Autodesk Inventor part; units mm, degrees
ref_plane "YZ Plane" through (0, 0, 0) normal (1, 0, 0) x (0, 1, 0)
ref_plane "XZ Plane" through (0, 0, 0) normal (0, 1, 0) x (-1, 0, 0)
ref_plane "XY Plane" through (0, 0, 0) normal (0, 0, 1) x (1, 0, 0)
sketch "Sketch1" plane through (0, 0, 0) normal (0, 0, 1) x (1, 0, 0)
  line L0 (-50, 45) -> (50, 45)
  line L1 (50, 45) -> (50, -45)
  line L2 (50, -45) -> (-50, -45)
  line L3 (-50, -45) -> (-50, 45)
  point P0 (0, 0)
  dimension "d0" = 100
  dimension "d1" = 90
  dimension "d2" = 50
  dimension "d3" = 45
extrude "Extrusion1" add sketch "Sketch1" along normal blind 2.6568
fillet "Fillet1" radius 10 4 edges at (50, 45, 1.3284) (-50, 45, 1.3284) (50, -45, 1.3284) (-50, -45, 1.3284)
sketch "Sketch2" plane through (0, 0, 2.6568) normal (0, 0, 1) x (1, 0, 0)
  line L0 (50, 35) -> (50, -35)
  line L1 (-40, 45) -> (40, 45)
  circle A0 centre (40, 32.3) radius 2.75
  circle A1 centre (40, -32.3) radius 3.5685
  point P0 (0, 0)
  dimension "d7" = 5.5
  dimension "d8" = 10
  dimension "d10" = 7.137
  dimension "d12" = 10
  dimension "d52" = 64.6
  dimension "d53" = 12.7
extrude "Extrusion2" cut sketch "Sketch2" against normal through all
pattern_linear "Rectangular Pattern1" count 3 spacing 40 along (-1, 0, 0) of "Extrusion2"
sketch "Sketch3" plane through (0, 0, 2.6568) normal (0, 0, 1) x (1, 0, 0)
  line L0 (40, -45) -> (-40, -45)
  line L1 (-50, -35) -> (-50, 35)
  circle A0 centre (-25, -10) radius 2.6
  point P0 (0, 0)
  dimension "d18" = 5.2
  dimension "d19" = 25
  dimension "d20" = 35
extrude "Extrusion3" cut sketch "Sketch3" against normal through all
pattern_linear "Rectangular Pattern2" count 3 spacing 25 along (1, 0, 0) count 2 spacing 20 along (0, 1, 0) of "Extrusion3"
properties part number "S2SM-01" material "Steel, Mild"
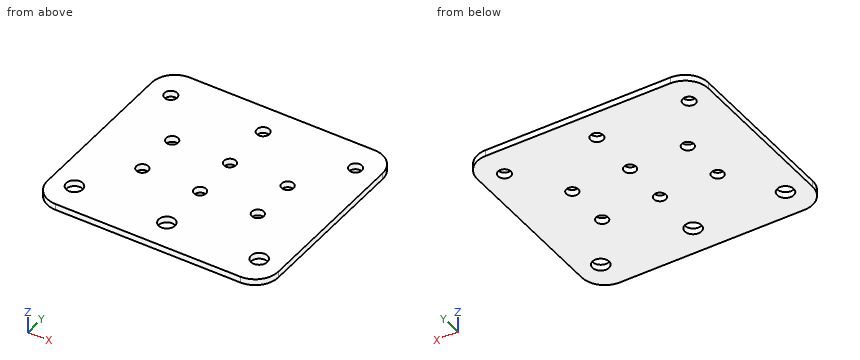
Work out the finished part from the listing and answer in its coordinate system (mm). Give positions to 0.01 mm unless a question says otherwise; leave off trailing zeros. Order: outer loops, then holes, each group sorted by start corner. A loop starts at its lowest first (then second) coordinate and runs counter-clockwise, first axis right, second up.
1. Section C-C, the plane z = 1.1 is taken. Give the number of separate pieces and of enclosed holes in the cut face, and give its area (3 significant figures).
Result sheet:
separate pieces: 1
enclosed holes: 12
area: 8,600 mm2
2. Straight lines are drawn through the part: L1, parallel to Y at x = -40, z = 1; L2, parallel to Y at x = 25, z = 2; L3, parallel to X at y = -35, z = 1.7. For each, find the intervals that lie inside material, in ascending order.
Result sheet:
L1: y = -45 to -35.87, -28.73 to 29.55, 35.05 to 45
L2: y = -45 to -12.6, -7.4 to 7.4, 12.6 to 45
L3: x = -50 to -42.33, -37.67 to -2.33, 2.33 to 37.67, 42.33 to 50
3. This flat-tipped pin is pushed along its axis until it touches: P1, Ø11.5, axis at x = 0, y = -32.3, coming from the -Z side. Where does it stop, or does it pass through?
Result sheet:
P1: stops at z = 0
4. Section D-D, the plane y = 32.3 is taken. Determine the outline of the cut face in (x, z), and give its area (3 significant figures).
Result sheet:
outline: (-50, 0) - (-42.75, 0) - (-42.75, 2.66) - (-50, 2.66) - close; (-37.25, 0) - (-2.75, 0) - (-2.75, 2.66) - (-37.25, 2.66) - close; (2.75, 0) - (37.25, 0) - (37.25, 2.66) - (2.75, 2.66) - close; (42.75, 0) - (50, 0) - (50, 2.66) - (42.75, 2.66) - close
area: 222 mm2
5. Section B-B, the plane y = 10 is taken. Determine the outline of the cut face in (x, z), and give its area (3 significant figures).
Result sheet:
outline: (-50, 0) - (-27.6, 0) - (-27.6, 2.66) - (-50, 2.66) - close; (-22.4, 0) - (-2.6, 0) - (-2.6, 2.66) - (-22.4, 2.66) - close; (2.6, 0) - (22.4, 0) - (22.4, 2.66) - (2.6, 2.66) - close; (27.6, 0) - (50, 0) - (50, 2.66) - (27.6, 2.66) - close
area: 224 mm2
6. Section A-A, the plane x = -25 is taken. Determine the outline of the cut face in (y, z), and give its area (3 significant figures).
Result sheet:
outline: (-45, 0) - (-12.6, 0) - (-12.6, 2.66) - (-45, 2.66) - close; (-7.4, 0) - (7.4, 0) - (7.4, 2.66) - (-7.4, 2.66) - close; (12.6, 0) - (45, 0) - (45, 2.66) - (12.6, 2.66) - close
area: 211 mm2
